Model file for the job. Use its own axes, mm. Face numbers are marked on the shaded views. A direction names the side the tool comes from. Give positions to 0.01 mm unless a question says otherwise; leave off trailing zeros. Write each loop counter-clockwise with the first axis right and the second up, starting at its lowest first coordinate (ties: lowest second). Pieces come first, ordered by that corner, then holes. Notation, with made-up numbers: (56, 9) - (105, 9) arc R13 cw to (105, 16) - close; hole circle Ø6 at (53.25, 28). An arc over 180 degrees is marked (long way). Use CSV: the item, a comma, the result in double quotes.
from build123d import *

# Parameters (mm, degrees)
SKETCH1_W          = 22
SKETCH1_H          = 28.5
FILLET1_R          = 4
SKETCH2_R          = 17.5
CUT_EXTRUDE1_DEPTH = 12
SKETCH3_R          = 17.5
CUT_EXTRUDE2_DEPTH = 8
SKETCH4_R          = 1.75
CUT_EXTRUDE3_DEPTH = 11


with BuildPart() as part:
    # Sketch1 → Revolve1 (revolve)
    with BuildSketch(Plane(origin=(0, 0, 0), x_dir=(1, 0, 0), z_dir=(0, 1, 0))):
        with Locations((0, 14.25)):
            Rectangle(SKETCH1_W, SKETCH1_H)
    revolve(axis=Axis((11, 0, 0), (-1, 0, 0)))

    # Fillet1
    fillet1_edges = [part.edges().sort_by_distance(p)[0] for p in [
        (11, 0, 28.5),
        (-11, 0, 28.5),
    ]]
    fillet(fillet1_edges, radius=FILLET1_R)

    # Sketch2 → Cut-Extrude1 (cut)
    with BuildSketch(Plane(origin=(11, 0, 0), x_dir=(0, 0, -1), z_dir=(1, 0, 0))):
        Circle(SKETCH2_R)
    extrude(amount=-CUT_EXTRUDE1_DEPTH, mode=Mode.SUBTRACT)

    # Sketch3 → Cut-Extrude2 (cut)
    with BuildSketch(Plane.ZY.offset(11)):
        Circle(SKETCH3_R)
    extrude(amount=-CUT_EXTRUDE2_DEPTH, mode=Mode.SUBTRACT)

    # Sketch4 → Cut-Extrude3 (cut, through all)
    with BuildSketch(Plane(origin=(-1, 0, 0), x_dir=(0, 0, -1), z_dir=(1, 0, 0))):
        Circle(SKETCH4_R)
    extrude(amount=-CUT_EXTRUDE3_DEPTH, mode=Mode.SUBTRACT)


solid = part.part
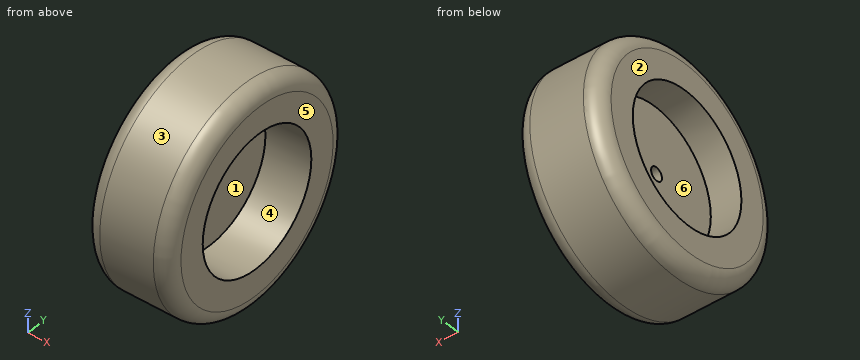
(1) Flat gauge pins, fed straight in: P1, Ø1, axis at x = -0.5, z = 0, coming from the +Y side; P2, Ø17.5, axis at y = -3.5, z = -3.5, coming from the -X side; P3, Ø4, axis at x = 3, z = 15.5, coming from the +Y side. Where does each tip first touch, or does it go through?
Checked values:
P1,"stops at y = 28.5"
P2,"stops at x = -3"
P3,"stops at y = 25.1"
(2) Saw through at D-D, the plane x = 8. List the corners of the cut face in (y, z).
Checked values:
outline,"circle Ø56.75 at (0, 0); hole circle Ø35 at (0, 0)"
(3) Pull direction Y, two halves, no side cores. Call the marked faces 1, 2 and 3: released by +Y, released by -Y, zero draft, split by the parting line, or undercut.
Checked values:
face 1,"undercut"
face 2,"zero draft"
face 3,"split by the parting line"
(4) Saw through at A-A, the plane y = 0. List the corners of the cut face in (x, z), then the cut area to 3 significant figures.
Checked values:
outline,"(-11, -24.5) arc R4 ccw to (-7, -28.5) - (7, -28.5) arc R4 ccw to (11, -24.5) - (11, -17.5) - (-1, -17.5) - (-1, -1.75) - (-3, -1.75) - (-3, -17.5) - (-11, -17.5) - close; (-11, 17.5) - (-3, 17.5) - (-3, 1.75) - (-1, 1.75) - (-1, 17.5) - (11, 17.5) - (11, 24.5) arc R4 ccw to (7, 28.5) - (-7, 28.5) arc R4 ccw to (-11, 24.5) - close"
area,"533 mm^2"
(5) Wall check: probe 1 along Y at (x, z) = (5.75, 0); probe 2 along X at (y, z) = (-8, -9.5); probe 3 along Y at (x, z) = (-4, 12.5). Give the ranges that are in metal, low to high. Write a range as [from, to].
Checked values:
probe 1,"y = [-28.5, -17.5], [17.5, 28.5]"
probe 2,"x = [-3, -1]"
probe 3,"y = [-25.61, -12.25], [12.25, 25.61]"
(6) Saw through at C-C, the plane x = -4.25. List the corners of the cut face in (y, z).
Checked values:
outline,"circle Ø57 at (0, 0); hole circle Ø35 at (0, 0)"
(7) 3-axis set-ups, long thin cutter, end or side, ignore diameter. For the marked faces 4, 5 and 6: which of +Z, -Z, +X, -X, +Y, -Y reach the whole face in a straight line?
Checked values:
face 4,"+X"
face 5,"+Z, -Z, +X, +Y, -Y"
face 6,"-X"
